from build123d import *

# Parameters (mm, degrees)
CROQUIS2_R              = 3
SALIENTE_EXTRUIR1_DEPTH = 5
SALIENTE_EXTRUIR2_DEPTH = 22.5
SALIENTE_EXTRUIR3_DEPTH = 5


with BuildPart() as part:
    # Croquis2 → Saliente-Extruir1 (new body)
    with BuildSketch(Plane(origin=(0, 0, 0), x_dir=(1, 0, 0), z_dir=(0, 1, 0))):
        with BuildLine():
            Line((7.5, -21.15), (5, 0))
            ThreePointArc((5, 0), (0, 5), (-5, 0))
            Line((-5, 0), (-9.15, 0))
            Line((-9.15, 0), (-9.15, -11.212351015))
            ThreePointArc((-9.15, -11.212351015), (-6.604850295, -17.877574723), (-0.264958583, -21.15))
            Line((-0.264958583, -21.15), (-0.127201334, -21.15))
            Line((-0.127201334, -21.15), (7.5, -21.15))
        make_face()
        with Locations(Location((0, 0, 0), (0, 0, 270))):
            Circle(CROQUIS2_R, mode=Mode.SUBTRACT)
    extrude(amount=SALIENTE_EXTRUIR1_DEPTH)

    # Croquis3 → Saliente-Extruir2 (add)
    with BuildSketch(Plane.XZ):
        Polygon((-9.15, 11.212351015), (6.325336999, 11.212351015), (5.855792624, 7.240005602), (-9.15, 7.240005602), align=None)
    extrude(amount=SALIENTE_EXTRUIR2_DEPTH)

    # Croquis4 → Saliente-Extruir3 (add)
    with BuildSketch(Plane.XZ.offset(22.5)):
        Polygon((5.855792624, 7.240005602), (6.325336999, 11.212351015), (-19.085175152, 11.212351015), (-19.085175152, 7.240005602), align=None)
    extrude(amount=SALIENTE_EXTRUIR3_DEPTH)


solid = part.part
Check sheet for the modelled part. Datum: model origin and axes. Units: mm. A direction names the side the tool comes from. Coordinates: 2 decimals unless noted, no trailing zeros. Write each loop counter-clockwise with the first axis right and the second up, starting at its lowest first coordinate (ties: lowest second). Pieces come first, ordered by that corner, then holes.
Item 1: Cross-section at B-B on x = -1.5. Record the boundary of the cut face in (y, z), then the cut area to 3 significant figures.
Numbers:
outline: (-27.5, 7.24) - (0, 7.24) - (0, 2.6) - (5, 2.6) - (5, 20.93) - (0, 20.93) - (0, 11.21) - (-27.5, 11.21) - close; (0, -4.77) - (5, -4.77) - (5, -2.6) - (0, -2.6) - close
area: 212 mm2
Item 2: Access from +Z, -Z, +X, -X, +Y, -Y to the whole of each face (thin tool, end or side, straight path). Record for faces 1 (the face through (-3, -14, 11.212)), 2 (the face through (-1, 5, 11)), 3 (the face through (-2, 0, 4)), 4 (the face through (4, 2, 21.15)), 5 (the face through (-14, -22.5, 9)).
Numbers:
face 1: +Z, +X, -X, -Y
face 2: +Z, -Z, +X, -X, +Y
face 3: -Z, +X, -X, -Y
face 4: +Z, +X, -X, +Y, -Y
face 5: +Z, -Z, -X, +Y
Item 3: Cross-section at C-C on z = 9.75. Record the boundary of the cut face in (x, y).
Numbers:
outline: (-19.09, -27.5) - (6.15, -27.5) - (6.15, 5) - (-9.15, 5) - (-9.15, -22.5) - (-19.09, -22.5) - close
Item 4: Cross-section at D-D on y = -11.5. Record the boundary of the cut face in (x, z).
Numbers:
outline: (-9.15, 7.24) - (5.86, 7.24) - (6.33, 11.21) - (-9.15, 11.21) - close
Item 5: Mould release check, pull along X, two halves, no side actions. Record for faces 6 (the face through (-9.15, -6, 8)), 7 (the face through (0.9, 2.46, 2.86)), 8 (the face through (-7, 2, 0)), 9 (the face through (0, 2, -5)): released by +X, released by -X, zero draft, split by the parting line, or undercut.
Numbers:
face 6: released by -X
face 7: undercut
face 8: zero draft
face 9: split by the parting line
Item 6: Cross-section at A-A on y = 3.5. Record the boundary of the cut face in (x, z), then the cut area to 3 significant figures.
Numbers:
outline: (-9.15, 0) - (-5, 0) arc R5 ccw to (5, 0) - (7.5, 21.15) - (-0.26, 21.15) arc R10 ccw to (-9.15, 11.21) - close; hole circle Ø6 at (0, 0)
area: 316 mm2
Item 7: Depth check by flat-ended pin: pin 1 Ø1.2 at (x, y) = (-7, 3.5) entering from -Z; pin 2 Ø11 at (x, z) = (-5, 15.5) entering from -Y; pin 3 Ø8 at (x, y) = (-1, -4.5) entering from -Z; pin 4 Ø2 at (x, y) = (2.5, -21) entering from +Z. Enter the tip coordinate at first touch or a pass-through.
Numbers:
pin 1: stops at z = 0
pin 2: stops at y = -27.5
pin 3: stops at z = 7.24
pin 4: stops at z = 11.21
Item 8: Scan lines: probe 1 along Z at (x, y) = (1, -13); probe 2 along Y at (x, z) = (5, 16.5); probe 3 along X at (y, z) = (-9, 9). Record each from-to range of solid material in increasing order.
Numbers:
probe 1: z = 7.24 to 11.21
probe 2: y = 0 to 5
probe 3: x = -9.15 to 6.06
